```python
from build123d import *

# Parameters (mm, degrees)
BOSS_EXTRU_1_DEPTH      = 45
ESQUISSE2_R             = 7
ENL_V_MAT_EXTRU_1_DEPTH = 45


with BuildPart() as part:
    # Esquisse1 → Boss.-Extru.1 (new body)
    with BuildSketch(Plane.XY):
        with BuildLine():
            Line((67.055498862, 42.585779817), (96.055498862, 42.585779817))
            Line((96.055498862, 42.585779817), (101.055498862, 37.585779817))
            Line((101.055498862, 37.585779817), (101.055498862, 18.585779817))
            Line((101.055498862, 18.585779817), (72.055498862, -16.414220183))
            Line((72.055498862, -16.414220183), (65.889453705, -16.414220183))
            ThreePointArc((65.889453705, -16.414220183), (61.82352383, -10.310269713), (59.418933012, -3.381493479))
            ThreePointArc((59.418933012, -3.381493479), (58.316949941, -0.102489997), (55.350190939, 1.676434271))
            Line((55.350190939, 1.676434271), (24.055498862, 1.676434271))
            Line((24.055498862, 1.676434271), (17.055498862, 8.676434271))
            Line((17.055498862, 8.676434271), (17.055498862, 26.676434271))
            Line((17.055498862, 26.676434271), (24.055498862, 33.676434271))
            Line((24.055498862, 33.676434271), (31.055498862, 33.676434271))
            Line((31.055498862, 33.676434271), (48.765077496, 30.553757741))
            ThreePointArc((48.765077496, 30.553757741), (59.817474753, 33.670568141), (67.055498862, 42.585779817))
        make_face()
    extrude(amount=BOSS_EXTRU_1_DEPTH)

    # Esquisse2 → Enlèv. mat.-Extru.1 (cut)
    with BuildSketch(Plane.XY.offset(45)):
        with Locations((31.055498862, 15.676434271)):
            Circle(ESQUISSE2_R)
    extrude(amount=-ENL_V_MAT_EXTRU_1_DEPTH, mode=Mode.SUBTRACT)


solid = part.part
```
Check sheet for the modelled part. Datum: model origin and axes. Units: mm. A direction names the side the tool comes from. Coordinates: 2 decimals unless noted, no trailing zeros. Write each loop counter-clockwise with the first axis right and the second up, starting at its lowest first coordinate (ties: lowest second). Pieces come first, ordered by that corner, then holes. Notation, with made-up numbers: M -20,51 L 22,51 A17 cw 22,70 Z; hole C 71,5.5 d7. An arc over 180 degrees is marked long. Write item = value, one per line. Start each with the question number.
1. Sectioned sample at B-B (z = 38.5). Record the cut outline in (x, y), then the cut area to 3 significant figures.
2. Mould release check, pull along Y, two halves, no side actions. Record for faces 6 (the flat face through (81, 42.586, 22)), 7 (the cylindrical face through (37.73, 17.78, 22.82)), 8 (the cylindrical face through (61.87, -10.4, 22.18)): pulls with the +Y half, pulls with the -Y half, needs draft (parallel to the pull), parting line crosses it, or undercut.
3. Sectioned sample at A-A (y = 14). Record the cut outline in (x, z), then the cut area to 3 significant figures.
4. Tool access check on faces 1 (the flat face through (101.055, 28, 22)), 2 (the flat face through (28, 33.676, 22)), 3 (the cylindrical face through (59.68, 33.58, 22.18)), 4 (the flat face through (69, -16.414, 22)), 5 (the flat face through (40, 1.676, 22)). Record the directions out of +Z, -Z, +X, -X, +Y, -Y that give a thin tool (end or side, any length) a straight path to the whole face; none if there is none.
5. Go/stop test with flat-tipped pins: pin 1 (12.5 mm diameter, centred on x = 31.06, y = 15.68, fed in from +Z); pin 2 (5 mm diameter, centred on x = 54, z = 37.5, fed in from +Y); pin 3 (10 mm diameter, centred on x = 60.5, y = 18.5, fed in from -Z); pin 4 (2 mm diameter, centred on x = 36, z = 29, fed in from +Y). Record where each tip stops, or that it passes through.
6. Sectioned sample at C-C (x = 35). Record the cut outline in (y, z).
7. Thickness scan on probe 1 along X at (y, z) = (21.5, 32); probe 2 along Y at (x, z) = (34, 32); probe 3 along Y at (x, z) = (47, 41). Record the ranges inside material, lowest first.
8. Sectioned sample at D-D (x = 57). Record the cut outline in (y, z).
The answers:
q1.outline = M 17.06,8.68 L 24.06,1.68 L 55.35,1.68 A5 cw 59.42,-3.38 A29 ccw 65.89,-16.41 L 72.06,-16.41 L 101.06,18.59 L 101.06,37.59 L 96.06,42.59 L 67.06,42.59 A19 cw 48.77,30.55 L 31.06,33.68 L 24.06,33.68 L 17.06,26.68 Z; hole C 31.06,15.68 d14
q1.area = 2,970 mm²
q2.face_6 = pulls with the +Y half
q2.face_7 = undercut
q2.face_8 = pulls with the -Y half
q3.outline = M 17.06,0 L 24.26,0 L 24.26,45 L 17.06,45 Z; M 37.85,0 L 97.26,0 L 97.26,45 L 37.85,45 Z
q3.area = 3,000 mm²
q4.face_1 = +Z, -Z, +X, +Y, -Y
q4.face_2 = +Z, -Z, -X, +Y
q4.face_3 = +Z, -Z, +Y
q4.face_4 = +Z, -Z, +X, -X, -Y
q4.face_5 = +Z, -Z, -X, -Y
q5.pin_1 = through
q5.pin_2 = 31.93
q5.pin_3 = 0
q5.pin_4 = 32.98
q6.outline = M 1.68,0 L 9.89,0 L 9.89,45 L 1.68,45 Z; M 21.46,0 L 32.98,0 L 32.98,45 L 21.46,45 Z
q7.probe_1 = 17.06 to 27.17, 34.94 to 101.06
q7.probe_2 = 1.68 to 9.33, 22.03 to 33.16
q7.probe_3 = 1.68 to 30.86
q8.outline = M 1.05,0 L 32.14,0 L 32.14,45 L 1.05,45 Z
